```python
from build123d import *

# Parameters (mm, degrees)
CROQUIS1_R                 = 40
CROQUIS1_R_2               = 30
SALIENTE_EXTRUIR1_DEPTH    = 90
CORTAR_EXTRUIR1_DEPTH      = 107.301458127
CORTAR_EXTRUIR1_DEPTH_BACK = 107.301458127
CROQUIS2_R                 = 5


with BuildPart() as part:
    # Croquis1 → Saliente-Extruir1 (new, symmetric)
    with BuildSketch(Plane(origin=(0, 0, 0), x_dir=(0, 0, -1), z_dir=(1, 0, 0))):
        with Locations(Location((0, 0, 0), (0, 0, 180))):
            Circle(CROQUIS1_R)
        with Locations(Location((0, 0, 0), (0, 0, 180))):
            Circle(CROQUIS1_R_2, mode=Mode.SUBTRACT)
    extrude(amount=SALIENTE_EXTRUIR1_DEPTH, both=True)

    # Croquis2 → Cortar-Extruir1 (cut, two sides: drawn at the far end of the back side and taken through both)
    with BuildSketch(Plane(origin=(0, 0, 0), x_dir=(1, 0, 0), z_dir=(0, 1, 0)).offset(-CORTAR_EXTRUIR1_DEPTH_BACK)):
        with Locations(Location((-80, 0, 0), (0, 0, 270))):
            Circle(CROQUIS2_R)
        with Locations(Location((80, 0, 0), (0, 0, 270))):
            Circle(CROQUIS2_R)
    extrude(amount=CORTAR_EXTRUIR1_DEPTH + CORTAR_EXTRUIR1_DEPTH_BACK, mode=Mode.SUBTRACT)


solid = part.part
```
Design review of the part built by this model. Coordinates are the model's own, in mm. Coordinates: 2 decimals unless noted, no trailing zeros. Order: outer loops, then holes, each group sorted by start corner. A loop starts at its lowest first (then second) coordinate and runs counter-clockwise, first axis right, second up.
1) Take a section at C-C, the plane x = 80. Give the boundary of the cut face in (y, z).
2) Mouldability with a two-part tool opening along Z and no side actions: class faces 1 (the cylindrical face through (-1.26, 29.287, -6.503)), 2 (the cylindrical face through (1.26, -1.76, -39.96)), 3 (the flat face through (90, -30, 6)) as +Z half, -Z half, draft (parallel to the pull), parting line (faces both ways), or undercut.
3) Take a section at B-B, the plane z = 0. Give the boundary of the cut face in (x, y), and give its area (3 significant figures).
4) Clearance check with flat-ended pins moving along their axes: pin 1 (1.5 mm diameter, centred on x = -67.5, y = 22.5, fed in from +Z); pin 2 (3 mm diameter, centred on x = -33.5, y = 24.5, fed in from -Z); pin 3 (6 mm diameter, centred on x = 38, y = 9, fed in from -Z). State where each tip first meets the part, or that it passes through.
5) Take a section at D-D, the plane x = -34. Give the boundary of the cut face in (y, z), and give its area (3 significant figures).
6) Wall thickness on line 1 along X through (y, z) = (-35, 0); line 2 along Y through (x, z) = (-31, 1); line 3 along Y through (x, z) = (34, -16): over which ranges is each line inside the solid? List them lowest first.
7) Take a section at A-A, the plane y = 0. Give the boundary of the cut face in (x, z).
Returned:
1. outline: (-39.69, -5) arc R40 ccw to (39.69, -5) - (29.58, -5) arc R30 cw to (-29.58, -5) - close; (-39.69, 5) - (-29.58, 5) arc R30 cw to (29.58, 5) - (39.69, 5) arc R40 ccw to start
2. face 1: undercut
2. face 2: parting line
2. face 3: draft
3. outline: (-90, -40) - (-85, -40) - (-85, -30) - (-90, -30) - close; (-90, 30) - (-85, 30) - (-85, 40) - (-90, 40) - close; (-75, -40) - (75, -40) - (75, -30) - (-75, -30) - close; (-75, 30) - (75, 30) - (75, 40) - (-75, 40) - close; (85, -40) - (90, -40) - (90, -30) - (85, -30) - close; (85, 30) - (90, 30) - (90, 40) - (85, 40) - close
3. area: 3,200 mm2
4. pin 1: stops at z = 33.57
4. pin 2: stops at z = -32.73
4. pin 3: stops at z = -39.55
5. outline: circle Ø80 at (0, 0); hole circle Ø60 at (0, 0)
5. area: 2,200 mm2
6. line 1: x = -90 to -85, -75 to 75, 85 to 90
6. line 2: y = -39.99 to -29.98, 29.98 to 39.99
6. line 3: y = -36.66 to -25.38, 25.38 to 36.66
7. outline: (-90, -40) - (90, -40) - (90, -30) - (-90, -30) - close; (-90, 30) - (90, 30) - (90, 40) - (-90, 40) - close
